Geometry: final body of the model. Coordinates: model frame, mm. A direction names the side the tool comes from. Coordinates: 2 decimals unless noted, no trailing zeros. Order: outer loops, then holes, each group sorted by start corner. A loop starts at its lowest first (then second) coordinate and runs counter-clockwise, first axis right, second up. Notation, with made-up numbers: M 79.5,29 L 103.5,29 A18 ccw 103.5,50 Z; hole C 31,-1.75 d11. An arc over 180 degrees is marked long. Use CSV: the item, a comma, the result in double quotes. Start each with the question number.
1. Section query D-D on z = 1. Return the cut outline in (x, y).
2. Material intervals for line 1 (X direction, y = 15.45, z = 5.9); line 2 (Z direction, x = -2.1, y = 15.2); line 3 (X direction, y = 8.5, z = 11.25), sorted ascending.
3. Set-up query: faces 1 (the flat face through (23.5, 9, 6)), 2 (the cylindrical face through (23.496, 21.824, 5.695)), 3 (the flat face through (-3.2, 16.4, 5.8)), 4 (the flat face through (0, 7, 6)), 5 (the flat face through (23.5, 18, 6)). Return all of +Z, -Z, +X, -X, +Y, -Y with unobstructed straight access to the full face (end or side cutting, diameter ignored); none if empty.
4. Section query B-B on x = 10.5. Return the cut outline in (y, z).
5. Section query A-A on x = 25.5. Return the cut outline in (y, z).
6. First-contact query: P1, Ø3, axis at y = 18, z = 3, coming from the +X side; P2, Ø1, axis at x = 5, z = 6.5, coming from the +Y side; P3, Ø2, axis at x = 26, z = 4, coming from the +Y side. Flat tips, straight axial feed; report the tip coordinate or a pass-through.
7. Section query C-C on y = 6. Return the cut outline in (x, z), and give its area (3 significant figures).
from build123d import *

# Parameters (mm, degrees)
DODANIE_WYCI_GNI_CIE1_DEPTH = 11.8
SZKIC2_R                    = 0.9
WYTNIJ_WYCI_GNI_CIE1_DEPTH  = 11.8
ZAOKR_GLENIE1_R             = 2
DODANIE_WYCI_GNI_CIE2_DEPTH = 3.7
SZKIC4_R                    = 1.9
DODANIE_WYCI_GNI_CIE3_DEPTH = 3.6


with BuildPart() as part:
    # Szkic1 → Dodanie-wyciągnięcie1 (new body)
    with BuildSketch(Plane.XY):
        Polygon((0, 0), (0, 14.8), (-4.4, 14.8), (-4.4, 16.4), (0, 16.4), (0, 20), (23.5, 20), (23.5, 16.4), (27.9, 16.4), (27.9, 14.8), (23.5, 14.8), (23.5, 2.5), (18.5, 0), align=None)
    extrude(amount=DODANIE_WYCI_GNI_CIE1_DEPTH)

    # Szkic2 → Wytnij-wyciągnięcie1 (cut)
    with BuildSketch(Plane(origin=(0, 16.4, 0), x_dir=(1, 0, 0), z_dir=(0, 1, 0))):
        with Locations((-2.1, -5.9)):
            Circle(SZKIC2_R)
        with Locations((25.6, -5.9)):
            Circle(SZKIC2_R)
    extrude(amount=-WYTNIJ_WYCI_GNI_CIE1_DEPTH, mode=Mode.SUBTRACT)

    # Zaokrąglenie1
    zaokr_glenie1_edges = [part.edges().sort_by_distance(p)[0] for p in [
        (-4.4, 15.6, 0),
        (27.9, 15.6, 0),
        (27.9, 15.6, 11.8),
        (-4.4, 15.6, 11.8),
    ]]
    fillet(zaokr_glenie1_edges, radius=ZAOKR_GLENIE1_R)

    # Szkic3 → Dodanie-wyciągnięcie2 (add)
    with BuildSketch(Plane(origin=(0, 20, 0), x_dir=(1, 0, 0), z_dir=(0, 1, 0))):
        with BuildLine():
            Line((11.85, -2.65), (12.164238784, -2.65))
            ThreePointArc((12.164238784, -2.65), (12.602449904, -2.548872079), (12.952030264, -2.265942029))
            ThreePointArc((12.952030264, -2.265942029), (23.5, -5.9), (12.952030264, -9.534057971))
            ThreePointArc((12.952030264, -9.534057971), (12.602449904, -9.251127921), (12.164238784, -9.15))
            Line((12.164238784, -9.15), (11.85, -9.15))
            ThreePointArc((11.85, -9.15), (8.6, -5.9), (11.85, -2.65))
        make_face()
    extrude(amount=DODANIE_WYCI_GNI_CIE2_DEPTH)

    # Szkic4 → Dodanie-wyciągnięcie3 (add)
    with BuildSketch(Plane(origin=(0, 23.7, 0), x_dir=(1, 0, 0), z_dir=(0, 1, 0))):
        with Locations((17.6, -5.9)):
            Circle(SZKIC4_R)
    extrude(amount=DODANIE_WYCI_GNI_CIE3_DEPTH)


solid = part.part
Results list:
1,outline,"M -4.13,14.8 L 0,14.8 L 0,0 L 18.5,0 L 23.5,2.5 L 23.5,14.8 L 27.63,14.8 L 27.63,16.4 L 23.5,16.4 L 23.5,20 L 20.89,20 L 20.89,23.7 L 14.31,23.7 L 14.31,20 L 0,20 L 0,16.4 L -4.13,16.4 Z"
2,line 1,"x = -4.4 to -3, -1.2 to 24.7, 26.5 to 27.9"
2,line 2,"z = 0 to 5, 6.8 to 11.8"
2,line 3,"x = 0 to 23.5"
3,face 1,"+Z, -Z, +X, -Y"
3,face 2,"+Y"
3,face 3,"+Z, -Z, -X, +Y"
3,face 4,"+Z, -Z, -X, -Y"
3,face 5,"+Z, -Z, +X, +Y"
4,outline,"M 0,0 L 20,0 L 20,2.94 L 23.7,2.94 L 23.7,8.86 L 20,8.86 L 20,11.8 L 0,11.8 Z"
5,outline,"M 14.8,0 L 16.4,0 L 16.4,5.01 L 14.8,5.01 Z; M 14.8,6.79 L 16.4,6.79 L 16.4,11.8 L 14.8,11.8 Z"
6,P1,"stops at x = 23.5"
6,P2,"stops at y = 20"
6,P3,"stops at y = 16.4"
7,outline,"M 0,0 L 23.5,0 L 23.5,11.8 L 0,11.8 Z"
7,area,"277 mm²"
